For this review, use the dimensioned drawing (mm, ordinates from the lowest corner) and the shaded views. Give positions to 0.01 mm unless a question says otherwise; leave off trailing zeros. Write each loop counter-clockwise with the first axis right and the second up, starting at its lowest first coordinate (ties: lowest second). Pieces come first, ordered by that corner, then holes. Notation, with made-up numbers: (78.5, 69) -> (127.5, 69) arc R19 cw to (127.5, 83) -> close; hole circle Ø11 at (61.5, -2). An arc over 180 degrees is marked (long way). Return JSON: item names as keys, results as strings.
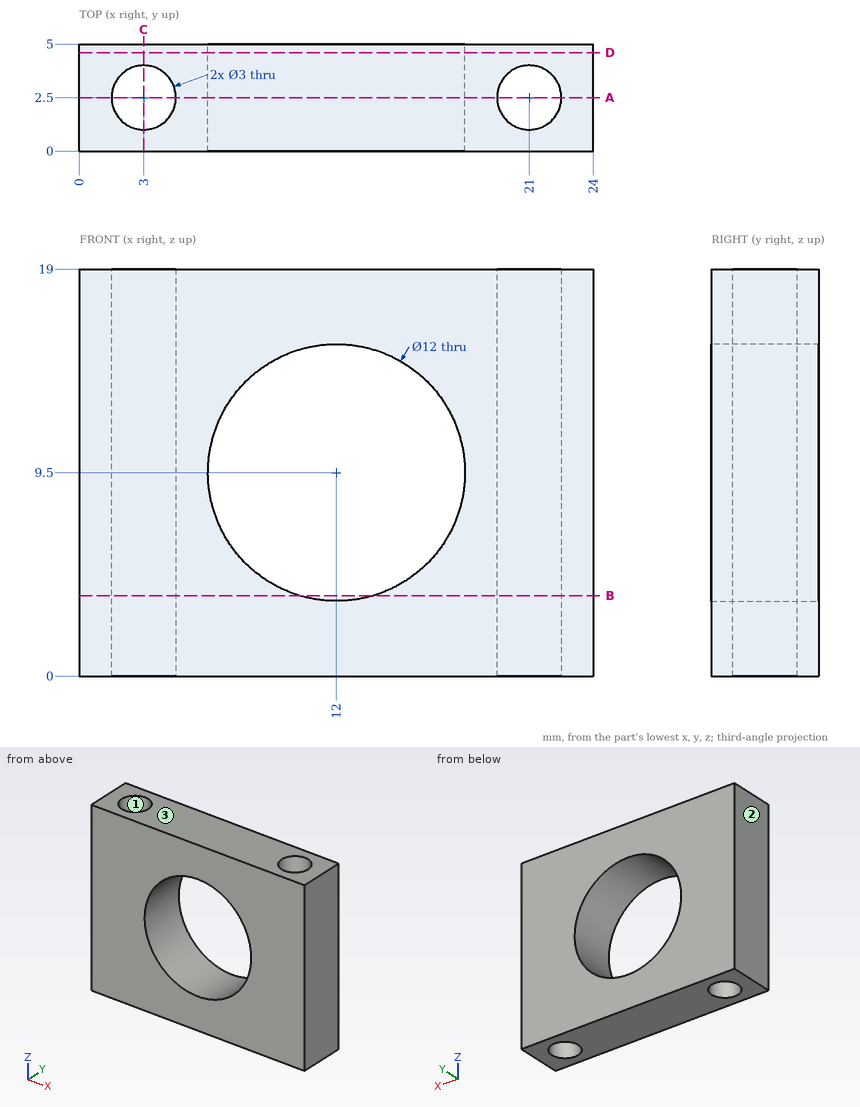
1. Add section C-C, the plane x = 3. State the section outline as (y, z) points, plus the area to 3 significant figures.
Results found:
{"outline": "(0, 0) -> (1, 0) -> (1, 19) -> (0, 19) -> close; (4, 0) -> (5, 0) -> (5, 19) -> (4, 19) -> close", "area": "38.0 mm²"}
2. The part is to be moulded in two halves that separate along X. For the marked faces 1, 2 and 3, say which applies: +X half, -X half, draft (parallel to the pull), parting line (faces both ways), or undercut.
Results found:
{"face 1": "undercut", "face 2": "-X half", "face 3": "draft"}
3. To check wall thickness, follow probe 1 along X at (y, z) = (2.4, 9.5); probe 2 along X at (y, z) = (2.25, 13.25); probe 3 along X at (y, z) = (1.55, 3). State the ranges of each line that lie inside material, in increasing order.
Results found:
{"probe 1": "x = 0 to 1.5, 4.5 to 6, 18 to 19.5, 22.5 to 24", "probe 2": "x = 0 to 1.52, 4.48 to 7.32, 16.68 to 19.52, 22.48 to 24", "probe 3": "x = 0 to 1.84, 4.16 to 19.84, 22.16 to 24"}
4. For pin 1 (2 mm diameter, centred on x = 14, z = 6.5, fed in from -Y), flat-tipped, find the tip position at first contact; note if it passes through.
Results found:
{"pin 1": "passes through"}
5. Add section B-B, the plane z = 3.75. State the section outline as (x, y) points.
Results found:
{"outline": "(0, 0) -> (10.29, 0) -> (10.29, 5) -> (0, 5) -> close; (13.71, 0) -> (24, 0) -> (24, 5) -> (13.71, 5) -> close; hole circle Ø3 at (3, 2.5); hole circle Ø3 at (21, 2.5)"}
6. Add section D-D, the plane y = 4.6. State the section outline as (x, z) points.
Results found:
{"outline": "(0, 0) -> (24, 0) -> (24, 19) -> (0, 19) -> close; hole circle Ø12 at (12, 9.5)"}
7. Add section A-A, the plane y = 2.5. State the section outline as (x, z) points, plus the area to 3 significant figures.
Results found:
{"outline": "(0, 0) -> (1.5, 0) -> (1.5, 19) -> (0, 19) -> close; (4.5, 0) -> (19.5, 0) -> (19.5, 19) -> (4.5, 19) -> close; (22.5, 0) -> (24, 0) -> (24, 19) -> (22.5, 19) -> close; hole circle Ø12 at (12, 9.5)", "area": "229 mm²"}
